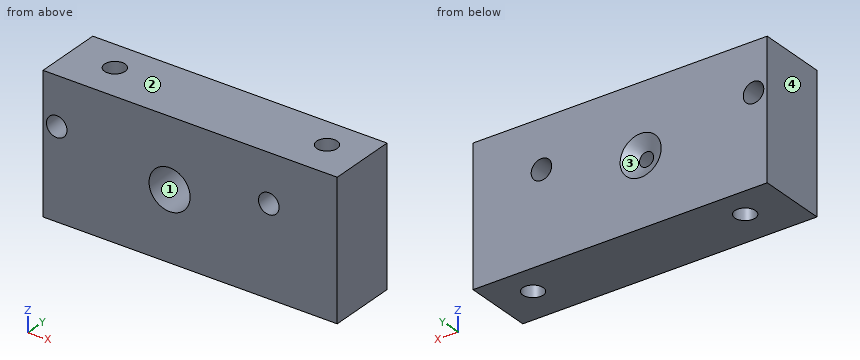
Autodesk Inventor part; units mm, degrees
ref_plane "YZ Plane" through (0, 0, 0) normal (1, 0, 0) x (0, 1, 0)
ref_plane "XZ Plane" through (0, 0, 0) normal (0, 1, 0) x (-1, 0, 0)
ref_plane "XY Plane" through (0, 0, 0) normal (0, 0, 1) x (1, 0, 0)
sketch "Sketch1" plane through (0, 0, 0) normal (0, 0, 1) x (1, 0, 0)
  line L0 (0, 0) -> (43, 0)
  line L1 (43, 0) -> (43, 10)
  line L2 (43, 10) -> (0, 10)
  line L3 (0, 10) -> (0, 0)
  circle A0 centre (6.5, 5.5) radius 1.5
  circle A1 centre (37.5, 5.5) radius 1.5
  dimension "d0" = 43
  dimension "d1" = 10
  dimension "d2" = 3
  dimension "d3" = 3
  dimension "d4" = 6.5
  dimension "d5" = 31
  dimension "d6" = 4.5
extrude "Extrusion1" add sketch "Sketch1" along normal blind 20
sketch "Sketch2" plane through (0, 10, 0) normal (0, 1, 0) x (1, 0, 0)
  line L0 (0, 0) -> (0, -20)
  line L1 (43, -20) -> (0, -20)
  circle A0 centre (2, -13) radius 1.5
  circle A1 centre (33, -13) radius 1.5
  dimension "d9" = 7
  dimension "d10" = 2
  dimension "d11" = 3
  dimension "d12" = 3
  dimension "d13" = 31
extrude "Extrusion2" cut sketch "Sketch2" against normal blind 20
sketch "Sketch3" plane through (0, 10, 0) normal (0, 1, 0) x (1, 0, 0)
  line L0 (0, 0) -> (0, -20)
  line L1 (43, -20) -> (0, -20)
  circle A0 centre (18.5, -10) radius 3
  dimension "d16" = 6
  dimension "d18" = 10
  dimension "d19" = 18.5
hole "Hole1" at (18.5, 10, 10) direction (0, -1, 0) diameter 6 depth 0.0001 tip angle 118
sketch "Sketch4" plane through (0, 0, 0) normal (0, -1, 0) x (1, 0, 0)
  line L0 (0, 20) -> (43, 20)
  line L1 (0, 0) -> (0, 20)
  circle A0 centre (18.5, 10) radius 2.2122
  dimension "d27" = 10
  dimension "d28" = 18.5
hole "Hole2" at (18.5, 0, 10) direction (0, 1, 0) diameter 6 depth 8 tip angle 135
thread "Thread1"
properties part number "heAluBase"
CAD build for the part. Positions are in the model's coordinates, mm. Face numbers are marked on the shaded views. Round coordinates to 2 decimals unless told otherwise and drop trailing zeros. Order: outer loops, then holes, each group sorted by start corner. A loop starts at its lowest first (then second) coordinate and runs counter-clockwise, first axis right, second up. Notation, with made-up numbers: (66.5, 43) -> (106.5, 43) arc R9 cw to (106.5, 58) -> close; hole circle Ø6 at (-26, -10.5). An arc over 180 degrees is marked (long way). Write item = value, one per line.
(1) Cut at B-B (y = 6.5). Write the cut outline in (x, z), plus the area to 3 significant figures.
Answers follow:
outline = (0, 0) -> (5.38, 0) -> (5.38, 20) -> (0, 20) -> close; (7.62, 0) -> (36.38, 0) -> (36.38, 20) -> (7.62, 20) -> close; (38.62, 0) -> (43, 0) -> (43, 20) -> (38.62, 20) -> close; hole circle Ø3 at (2, 13); hole circle Ø6 at (18.5, 10); hole circle Ø3 at (33, 13)
area = 728 mm²
(2) Pull direction Z, two halves, no side cores. Call the marked faces 1, 2, 3 and 4: +Z half, -Z half, draft (parallel to the pull), parting line (faces both ways), or undercut.
Answers follow:
face_1 = undercut
face_2 = +Z half
face_3 = undercut
face_4 = draft
(3) Flat gauge pin, fed straight in: P1, Ø5.5, axis at x = 18.5, z = 10, coming from the +Y side. Where does the tip first touch, or does it go through?
Answers follow:
P1 = 9.85
(4) Cut at A-A (x = 37.5). Write the cut outline in (y, z), plus the area to 3 significant figures.
Answers follow:
outline = (0, 0) -> (4, 0) -> (4, 20) -> (0, 20) -> close; (7, 0) -> (10, 0) -> (10, 20) -> (7, 20) -> close
area = 140 mm²
(5) Cut at C-C (z = 10). State how many separate pieces and enclosed holes the cut face has, plus the area to 3 significant figures.
Answers follow:
separate_pieces = 2
enclosed_holes = 2
area = 360 mm²
(6) Cut at D-D (z = 5.25). Write the cut outline in (x, y).
Answers follow:
outline = (0, 0) -> (43, 0) -> (43, 10) -> (0, 10) -> close; hole circle Ø3 at (6.5, 5.5); hole circle Ø3 at (37.5, 5.5)
(7) Drill centre lines: L1, parallel to Y at x = 37.5, z = 13; L2, parallel to Z at x = 33, y = 5; L3, parallel to X at y = 4.5, z = 13.25. Where is each one in solid material? Low to high.
Answers follow:
L1 = 0 to 4, 7 to 10
L2 = 0 to 11.5, 14.5 to 20
L3 = 0 to 0.52, 3.48 to 5.38, 7.62 to 31.52, 34.48 to 36.38, 38.62 to 43
